from build123d import *

# Parameters (mm, degrees)
F0_R     = 20
F0_R_2   = 12.75
F1_DEPTH = 100
F3_DEPTH = 25
F4_W     = 2
F4_H     = 2
F5_DEPTH = 50


with BuildPart() as f1:
    # F0 (on Top) → F1 (new body, symmetric)
    with BuildSketch(Plane.XY):
        Circle(F0_R)
        Circle(F0_R_2, mode=Mode.SUBTRACT)
    extrude(amount=F1_DEPTH, both=True)

    # F2 (on Right) → F3 (intersect, symmetric)
    with BuildSketch(Plane.YZ):
        Polygon((-5, 65.33519), (-30, 65.33519), (-30, -64.66481), (-5, -64.66481), (-5, -74.66481), (5, -74.66481), (5, -64.66481), (30, -64.66481), (30, 65.33519), (5, 65.33519), (5, 55.33519), (-5, 55.33519), align=None)
    extrude(amount=F3_DEPTH, both=True, mode=Mode.INTERSECT)

    # F4 (on Top) → F5 (cut, symmetric)
    with BuildSketch(Plane.XY):
        with Locations((0, 12.75)):
            Rectangle(F4_W, F4_H)
        Polygon((-6.09746, 10.093735), (-7.27303, 11.711769), (-8.891064, 10.536198), (-7.715494, 8.918164), align=None)
        Polygon((-10.865897, 4.582006), (-12.76801, 5.20004), (-13.386044, 3.297927), (-11.483931, 2.679893), align=None)
        Polygon((-11.483931, -2.679893), (-13.386044, -3.297927), (-12.76801, -5.20004), (-10.865897, -4.582006), align=None)
        Polygon((-7.715494, -8.918164), (-8.891064, -10.536198), (-7.27303, -11.711769), (-6.09746, -10.093735), align=None)
        with Locations((0, -12.75)):
            Rectangle(F4_W, F4_H)
        Polygon((6.09746, -10.093735), (7.27303, -11.711769), (8.891064, -10.536198), (7.715494, -8.918164), align=None)
        Polygon((10.865897, -4.582006), (12.76801, -5.20004), (13.386044, -3.297927), (11.483931, -2.679893), align=None)
        Polygon((11.483931, 2.679893), (13.386044, 3.297927), (12.76801, 5.20004), (10.865897, 4.582006), align=None)
        Polygon((7.715494, 8.918164), (8.891064, 10.536198), (7.27303, 11.711769), (6.09746, 10.093735), align=None)
    extrude(amount=F5_DEPTH, both=True, mode=Mode.SUBTRACT)


solid = f1.part
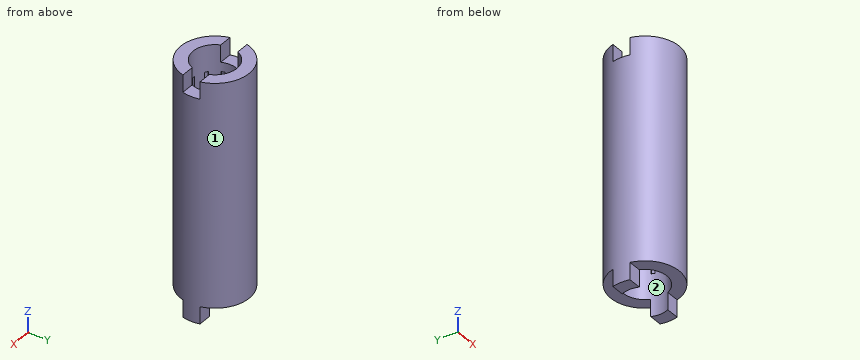
Input: part model. Units: mm. Frame: model coordinates. Face numbers are marked on the shaded views. Give positions to 0.01 mm unless a question says otherwise; leave off trailing zeros. Write each loop counter-clockwise with the first axis right and the second up, starting at its lowest first coordinate (ties: lowest second). Pieces come first, ordered by that corner, then holes.
Q1. Section C-C, the plane z = -54. Output: boundary loops of the cut face in (x, y).
Q2. Section D-D, the plane x = 16. Output: boundary loops of the cut face in (y, z).
Q3. Section B-B, the plane x = 3. Output: boundary loops of the cut face in (y, z), plus the area to 3 significant figures.
Q4. Section A-A, the plane y = 0. Output: boundary loops of the cut face in (x, z).
Q5. Material intervals for probe 1 along Y at (x, z) = (0, 6); probe 2 along X at (y, z) = (11, 43.5); probe 3 along X at (y, z) = (0, -32), sorted ascending.
Q6. First-contact query: P1, Ø5, axis at x = 3, z = -40.5, coming from the -Y side; P2, Ø2.5, axis at x = 16, z = -67.5, coming from the +Y side; P3, Ø5, axis at y = -15.5, z = 27, coming from the -X side; P4, Ø6, axis at x = 3, y = 9, coming from the +Z side. Flat tips, straight axial feed; report the tip coordinate or a pass-through.
Q7. Pull-direction query (X, two-part tool) for the marked faces 1 and 2; classes: pulls with the +X half, pulls with the -X half, needs draft (parallel to the pull), parting line crosses it, or undercut.
Filled in:
1. outline: circle Ø40 at (0, 0); hole circle Ø25.5 at (0, 0)
2. outline: (-12, -64.66) - (-5, -64.66) - (-5, -74.66) - (5, -74.66) - (5, -64.66) - (12, -64.66) - (12, 65.34) - (5, 65.34) - (5, 55.34) - (-5, 55.34) - (-5, 65.34) - (-12, 65.34) - close
3. outline: (-19.77, -64.66) - (-12.39, -64.66) - (-12.39, 65.34) - (-19.77, 65.34) - close; (12.39, -64.66) - (19.77, -64.66) - (19.77, 65.34) - (12.39, 65.34) - close
3. area: 1,920 mm2
4. outline: (-20, -74.66) - (-12.75, -74.66) - (-12.75, 55.34) - (-20, 55.34) - close; (12.75, -74.66) - (20, -74.66) - (20, 55.34) - (12.75, 55.34) - close
5. probe 1: y = -20 to -13.75, 13.75 to 20
5. probe 2: x = -16.7 to -8.25, -6.76 to -6.45, 6.45 to 6.76, 8.25 to 16.7
5. probe 3: x = -20 to -12.75, 12.75 to 20
6. P1: stops at y = -19.99
6. P2: stops at y = 5
6. P3: stops at x = -15.2
6. P4: passes through
7. face 1: parting line crosses it
7. face 2: undercut
